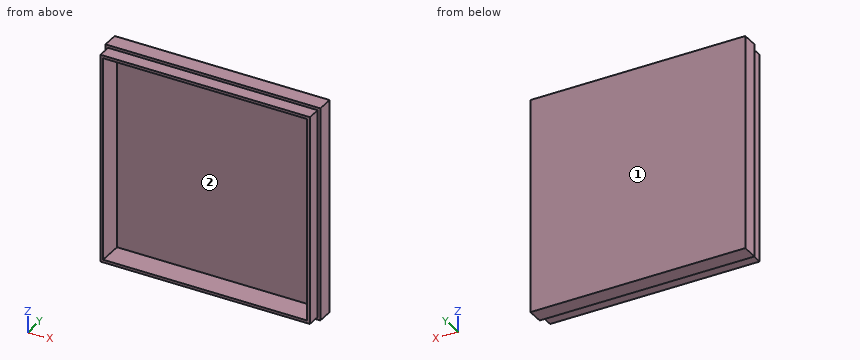
```python
from build123d import *

# Parameters (mm, degrees)
SKETCH_1_W          = 39
SKETCH_1_H          = 39
EXTRUDE_1_DEPTH     = 5.5
SKETCH_2_W          = 39
SKETCH_2_H          = 3
EXTRUDE_2_DEPTH     = 0.5
SKETCH_3_W          = 39.5
SKETCH_3_H          = 3
EXTRUDE_3_DEPTH     = 0.5
SKETCH_5_W          = 39.5
SKETCH_5_H          = 3
EXTRUDE_4_DEPTH     = 0.5
SKETCH_6_W          = 40
SKETCH_6_H          = 3
EXTRUDE_5_DEPTH     = 0.5
SKETCH_7_W          = 38
SKETCH_7_H          = 38
CUT_EXTRUDE_1_DEPTH = 4.5


with BuildPart() as part:
    # Эскиз1 → Бобышка-Вытянуть1 (new body)
    with BuildSketch(Plane(origin=(0, 0, 0), x_dir=(1, 0, 0), z_dir=(0, 1, 0))):
        with Locations((2.720930233, -12.848837209)):
            Rectangle(SKETCH_1_W, SKETCH_1_H)
    extrude(amount=EXTRUDE_1_DEPTH)

    # Эскиз2 → Бобышка-Вытянуть2 (add)
    with BuildSketch(Plane.ZY.offset(16.779069767)):
        with Locations((12.848837209, 4)):
            Rectangle(SKETCH_2_W, SKETCH_2_H)
    extrude(amount=EXTRUDE_2_DEPTH)

    # Эскиз3 → Бобышка-Вытянуть3 (add)
    with BuildSketch(Plane.XY.offset(32.348837209)):
        with Locations((2.470930233, 4)):
            Rectangle(SKETCH_3_W, SKETCH_3_H)
    extrude(amount=EXTRUDE_3_DEPTH)

    # Эскиз5 → Бобышка-Вытянуть4 (add)
    with BuildSketch(Plane(origin=(22.220930233, 0, 0), x_dir=(0, 0, -1), z_dir=(1, 0, 0))):
        with Locations((-13.098837209, 4)):
            Rectangle(SKETCH_5_W, SKETCH_5_H)
    extrude(amount=EXTRUDE_4_DEPTH)

    # Эскиз6 → Бобышка-Вытянуть5 (add)
    with BuildSketch(Plane(origin=(0, 0, -6.651162791), x_dir=(-1, 0, 0), z_dir=(0, 0, -1))):
        with Locations((-2.720930233, 4)):
            Rectangle(SKETCH_6_W, SKETCH_6_H)
    extrude(amount=EXTRUDE_5_DEPTH)

    # Эскиз7 → Вырез-Вытянуть1 (cut)
    with BuildSketch(Plane.XZ):
        with Locations((2.720930233, 12.848837209)):
            Rectangle(SKETCH_7_W, SKETCH_7_H)
    extrude(amount=-CUT_EXTRUDE_1_DEPTH, mode=Mode.SUBTRACT)


solid = part.part
```
Model file for the job. Use its own axes, mm. Face numbers are marked on the shaded views. Coordinates: 2 decimals unless noted, no trailing zeros. Order: outer loops, then holes, each group sorted by start corner. A loop starts at its lowest first (then second) coordinate and runs counter-clockwise, first axis right, second up. Notation, with made-up numbers: (3.25, 57.5) -> (58.25, 57.5) arc R14 ccw to (58.25, 72.5) -> close; hole circle Ø6 at (18.5, 40). An arc over 180 degrees is marked (long way). Return JSON: item names as keys, results as strings.
Item 1: Pin check, flat tips, straight feed: P1, Ø11.5, axis at x = -3, z = 7.5, coming from the -Y side; P2, Ø2, axis at y = 1, z = 14, coming from the +X side; P3, Ø1.2, axis at x = 11.5, y = 1.5, coming from the +Z side; P4, Ø3, axis at x = -7, y = 1.5, coming from the -Z side. Stop position of each tip, or through.
Model answer:
{"P1": "stops at y = 4.5", "P2": "stops at x = 22.22", "P3": "stops at z = 32.35", "P4": "stops at z = -7.15"}
Item 2: Slice it at C-C (z = 8.5). Write the cut outline in (x, y).
Model answer:
{"outline": "(-17.28, 2.5) -> (-16.78, 2.5) -> (-16.78, 0) -> (-16.28, 0) -> (-16.28, 4.5) -> (21.72, 4.5) -> (21.72, 0) -> (22.22, 0) -> (22.22, 2.5) -> (22.72, 2.5) -> (22.72, 5.5) -> (-17.28, 5.5) -> close"}
Item 3: Mould opens along Z. For the marked faces 1 and 2 say: pulls with the +Z half, pulls with the -Z half, needs draft (parallel to the pull), parting line crosses it, or undercut.
Model answer:
{"face 1": "needs draft", "face 2": "undercut"}
Item 4: Slice it at B-B (x = -8). Write the cut outline in (y, z).
Model answer:
{"outline": "(0, -6.65) -> (2.5, -6.65) -> (2.5, -7.15) -> (5.5, -7.15) -> (5.5, 32.85) -> (2.5, 32.85) -> (2.5, 32.35) -> (0, 32.35) -> (0, 31.85) -> (4.5, 31.85) -> (4.5, -6.15) -> (0, -6.15) -> close"}
Item 5: Wall check: line 1 along Z through (x, y) = (-12, 1.55); line 2 along X through (y, z) = (1.15, 17.5); line 3 along Z through (x, y) = (13, 3.55). Give the ranges that are in metal, low to high. Write a range as from..to.
Model answer:
{"line 1": "z = -6.65..-6.15, 31.85..32.35", "line 2": "x = -16.78..-16.28, 21.72..22.22", "line 3": "z = -7.15..-6.15, 31.85..32.85"}
Item 6: Slice it at A-A (y = 1.8). Write the cut outline in (x, z), then the cut area to 3 significant figures.
Model answer:
{"outline": "(-16.78, -6.65) -> (22.22, -6.65) -> (22.22, 32.35) -> (-16.78, 32.35) -> close; hole (-16.28, -6.15) -> (21.72, -6.15) -> (21.72, 31.85) -> (-16.28, 31.85) -> close", "area": "77.0 mm²"}
